Here's how the part is built. I have some questions about the finished solid (model axes, mm). Face numbers are marked on the shaded views. A direction names the side the tool comes from. Coordinates: 2 decimals unless noted, no trailing zeros. Loops run counter-clockwise (first coordinate to the right, second up) from the corner with the lowest first, then second, coordinate; pieces in that order, holes last.
```python
from build123d import *

# Parameters (mm, degrees)
F0_W     = 25
F0_H     = 27
F0_R     = 1.25
F0_R_2   = 7.75
F1_DEPTH = 3
F0_H_2   = 3
F2_DEPTH = 40
F3_R     = 4
F4_DEPTH = 25
F5_R     = 1


with BuildPart() as f1:
    # F0 (on Top) → F1 (new body)
    with BuildSketch(Plane.XY):
        with Locations((0, -1.5)):
            Rectangle(F0_W, F0_H)
        with Locations((-10, -2)):
            Circle(F0_R, mode=Mode.SUBTRACT)
        with Locations((0, -2)):
            Circle(F0_R_2, mode=Mode.SUBTRACT)
    extrude(amount=F1_DEPTH)

    # F0 (on Top) → F2 (join)
    with BuildSketch(Plane.XY):
        with Locations((0, 13.5)):
            Rectangle(F0_W, F0_H_2)
    extrude(amount=F2_DEPTH)

    # F3 (on face) → F4 (cut)
    with BuildSketch(Plane(origin=(0, 15, 0), x_dir=(-1, 0, 0), z_dir=(0, 1, 0))):
        with Locations((0, 20)):
            Circle(F3_R)
    extrude(amount=-F4_DEPTH, mode=Mode.SUBTRACT)

    # F5
    f5_edges = [f1.edges().sort_by_distance(p)[0] for p in [
        (12.5, -15, 1.5),
        (-12.5, -15, 1.5),
    ]]
    fillet(f5_edges, radius=F5_R)


solid = f1.part
```
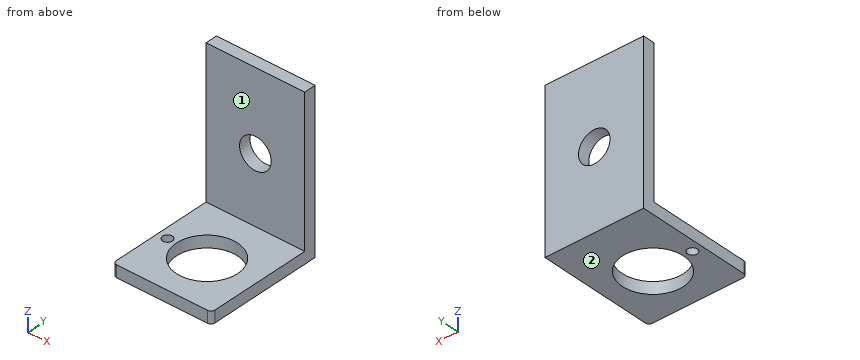
1. I want a section at C-C (x = 0). Please give me the cut outline in (y, z), then the cut area to 4 significant figures.
2. On a 3-axis mill with a long thin cutter (end or side, diameter ignored), from which of +Z, -Z, +X, -X, +Y, -Y can I reach the whole of each face in a straight line? I mean the marked faces 1 and 2. Say none if no direction works.
3. I need wall thicknesses on line 1 along Z through (x, y) = (0, 13.6); line 2 along Z through (x, y) = (5, 6.75); line 3 along Y through (x, z) = (7, 5). Which ranges of each line are inside material? Lowest first, please.
4. For pin 1 (9 mm diameter, centred on x = 0, z = 20, fed in from -Y); pin 2 (7.5 mm diameter, centred on x = 4.5, y = 5, fed in from +Z), each with a flat end and sliding along its axis, tell me the tip position at first contact or that it passes through.
5. I want a section at D-D (z = 20). Please give me the cut outline in (x, y), then the cut area to 3 significant figures.
6. I want a section at A-A (y = -2). Please give me the cut outline in (x, z), then the cut area to 3 significant figures.
7. I want a section at B-B (z = 2). Please give me the cut outline in (x, y).
Response values:
1. outline: (-15, 0) - (-9.75, 0) - (-9.75, 3) - (-15, 3) - close; (5.75, 0) - (15, 0) - (15, 16) - (12, 16) - (12, 3) - (5.75, 3) - close; (12, 24) - (15, 24) - (15, 40) - (12, 40) - close
1. area: 130.5 mm2
2. face 1: +Z, +X, -X, -Y
2. face 2: -Z, +X, -X, +Y, -Y
3. line 1: z = 0 to 16, 24 to 40
3. line 2: z = 0 to 3
3. line 3: y = 12 to 15
4. pin 1: stops at y = 12
4. pin 2: stops at z = 3
5. outline: (-12.5, 12) - (-4, 12) - (-4, 15) - (-12.5, 15) - close; (4, 12) - (12.5, 12) - (12.5, 15) - (4, 15) - close
5. area: 51.0 mm2
6. outline: (-12.5, 0) - (-11.25, 0) - (-11.25, 3) - (-12.5, 3) - close; (-8.75, 0) - (-7.75, 0) - (-7.75, 3) - (-8.75, 3) - close; (7.75, 0) - (12.5, 0) - (12.5, 3) - (7.75, 3) - close
6. area: 21.0 mm2
7. outline: (-12.5, -14) arc R1 ccw to (-11.5, -15) - (11.5, -15) arc R1 ccw to (12.5, -14) - (12.5, 15) - (-12.5, 15) - close; hole circle Ø2.5 at (-10, -2); hole circle Ø15.5 at (0, -2)
